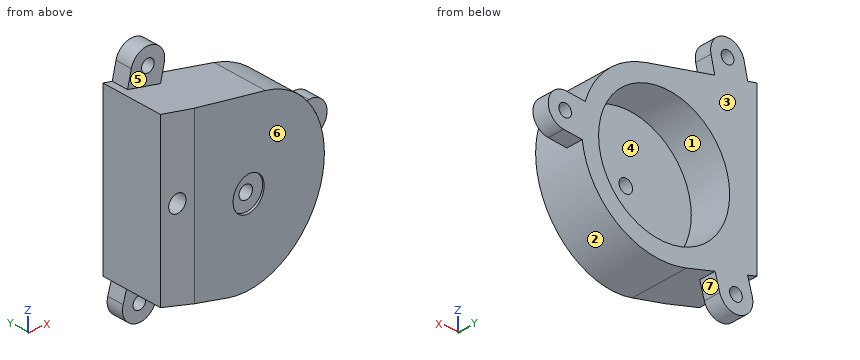
```python
from build123d import *

# Parameters (mm, degrees)
SKETCH1_R               = 15.5
BOSS_EXTRUDE1_DEPTH     = 5
SKETCH2_R               = 15.5
BOSS_EXTRUDE2_DEPTH     = 15
CUT_EXTRUDE7_DEPTH      = 26
CUT_EXTRUDE7_DEPTH_BACK = 20.5
SKETCH18_R              = 1.6
CUT_EXTRUDE8_DEPTH      = 6
SKETCH19_R              = 2.05
CUT_EXTRUDE9_DEPTH      = 6
CUT_EXTRUDE10_REACH     = 4
SKETCH20_R              = 4
SKETCH21_R              = 1.5
SKETCH21_R_2            = 4
BOSS_EXTRUDE3_DEPTH     = 4


with BuildPart() as part:
    # Sketch1 → Boss-Extrude1 (new body)
    with BuildSketch(Plane(origin=(0, 0, 0), x_dir=(1, 0, 0), z_dir=(0, 1, 0))):
        Circle(SKETCH1_R)
    extrude(amount=BOSS_EXTRUDE1_DEPTH)

    # Sketch2 → Boss-Extrude2 (add)
    with BuildSketch(Plane.XZ):
        with BuildLine():
            Line((-22, -14), (-5.351429285, -18.751325409))
            ThreePointArc((-5.351429285, -18.751325409), (18.889988887, -4.839247858), (4.323483194, 19.014665211))
            Line((4.323483194, 19.014665211), (-22, 25))
            Line((-22, 25), (-22, -14))
        make_face()
        Circle(SKETCH2_R, mode=Mode.SUBTRACT)
    extrude(amount=-BOSS_EXTRUDE2_DEPTH)

    # Sketch17 → Cut-Extrude7 (cut, two sides)
    with BuildSketch(Plane.XY) as cut_extrude7_sk:
        Polygon((19.5, 0), (-14, 0), (19.5, 3), align=None)
    extrude(amount=CUT_EXTRUDE7_DEPTH, mode=Mode.SUBTRACT)
    extrude(cut_extrude7_sk.sketch, amount=-CUT_EXTRUDE7_DEPTH_BACK, mode=Mode.SUBTRACT)

    # Sketch18 → Cut-Extrude8 (cut, through all)
    with BuildSketch(Plane(origin=(0, 5, 0), x_dir=(1, 0, 0), z_dir=(0, 1, 0))):
        Circle(SKETCH18_R)
    extrude(amount=-CUT_EXTRUDE8_DEPTH, mode=Mode.SUBTRACT)

    # Sketch19 → Cut-Extrude9 (cut)
    with BuildSketch(Plane.XZ):
        with Locations((-18, 5.5)):
            Circle(SKETCH19_R)
    extrude(amount=-CUT_EXTRUDE9_DEPTH, mode=Mode.SUBTRACT)

    # Sketch20 → Cut-Extrude10 (cut, up to next)
    with BuildSketch(Plane(origin=(0, 2, 0), x_dir=(1, 0, 0), z_dir=(0, 1, 0)), mode=Mode.PRIVATE) as cut_extrude10_sk1:
        Circle(SKETCH20_R)
    cut_extrude10_tool1 = extrude(cut_extrude10_sk1.sketch, amount=-CUT_EXTRUDE10_REACH, mode=Mode.PRIVATE) & part.part
    add(cut_extrude10_tool1.solids().sort_by_distance((0, 2, 0))[0], mode=Mode.SUBTRACT)

    # Sketch21 → Boss-Extrude3 (add)
    with BuildSketch(Plane(origin=(0, 15, 0), x_dir=(1, 0, 0), z_dir=(0, 1, 0))):
        with BuildLine():
            ThreePointArc((-13.153574275, 20.684381981), (-18.097729084, 23.433078622), (-20.846425725, 18.488923813))
            Line((-20.846425725, 18.488923813), (-19.748696641, 14.642498088))
            Line((-19.748696641, 14.642498088), (-12.055845191, 16.837956256))
            Line((-12.055845191, 16.837956256), (-13.153574275, 20.684381981))
        make_face()
        with Locations((-17, 19.586652897)):
            Circle(SKETCH21_R, mode=Mode.SUBTRACT)
        with BuildLine():
            Line((-11.099555854, -26.623594872), (-11.986424202, -22.723150726))
            Line((-11.986424202, -22.723150726), (-19.787312493, -24.496887421))
            Line((-19.787312493, -24.496887421), (-18.900444146, -28.397331567))
            ThreePointArc((-18.900444146, -28.397331567), (-14.113131653, -31.410907365), (-11.099555854, -26.623594872))
        make_face()
        with Locations((-15, -27.51046322)):
            Circle(SKETCH21_R, mode=Mode.SUBTRACT)
        with BuildLine():
            ThreePointArc((23.061952434, -6.032938747), (20.346397625, -4.619310384), (19.425796615, -1.699536959))
            ThreePointArc((19.425796615, -1.699536959), (19.147003171, -3.69354431), (18.664086253, -5.648175312))
            Line((18.664086253, -5.648175312), (23.061952434, -6.032938747))
        make_face()
        with Locations((23.410575405, -2.048159955)):
            Circle(SKETCH21_R_2)
        with Locations((23.410575405, -2.048159955)):
            Circle(SKETCH21_R, mode=Mode.SUBTRACT)
        with BuildLine():
            Line((23.759198376, 1.936618838), (19.361332194, 2.321382272))
            ThreePointArc((19.361332194, 2.321382272), (19.497494408, 0.31258889), (19.425796615, -1.699536959))
            ThreePointArc((19.425796615, -1.699536959), (20.839424976, 1.016017826), (23.759198376, 1.936618838))
        make_face()
    extrude(amount=-BOSS_EXTRUDE3_DEPTH)


solid = part.part
```
The model under review builds one solid part; all positions refer to its coordinate system, in mm. Face numbers are marked on the shaded views. A direction names the side the tool comes from. Give positions to 0.01 mm unless a question says otherwise; leave off trailing zeros. Write each loop counter-clockwise with the first axis right and the second up, starting at its lowest first coordinate (ties: lowest second). Pieces come first, ordered by that corner, then holes.
(1) The part is to be moulded in two halves that separate along Z. For the marked faces 1, 2, 3 and 4, say which applies: released by +Z, released by -Z, zero draft, split by the parting line, or undercut.
(2) To check wall thickness, follow L1, parallel to X at y = 13.25, z = 2; L2, parallel to X at y = 10.5, z = -3; L3, parallel to Z at x = 0, y = 3.35. State the ranges of each line that lie inside material, in increasing order.
(3) Consider section A-A, the plane y = 7.25. Give the boundary of the cut face in (x, z), and give its area (3 significant figures).
(4) Consider section C-C, the plane x = 3. Give the boundary of the cut face in (y, z), and give its area (3 significant figures).
(5) Tool access review of the marked faces 5, 6 and 7: name each direction out of +Z, -Z, +X, -X, +Y, -Y from which nothing blocks a thin tool from reaching the whole face with its end or side.
(6) Consider section B-B, the plane y = 3.75. Give the boundary of the cut face in (x, z).
(7) Consider section D-D, the plane x = 8.5. Give the boundary of the cut face in (y, z), and give its area (3 significant figures).
(8) For P1, Ø3, axis at x = 11.5, z = 19.5, coming from the +Y side; P2, Ø1, axis at x = 10.5, y = 5, coming from the +Z side; P3, Ø4, axis at x = 0, z = 0, coming from the -Y side; P4, Ø4, axis at x = 18, y = 2, coming from the -Z side, all flat-tipped, find the tip position at first contact; note any pin that passes through.
Returned:
1. face 1: undercut
1. face 2: split by the parting line
1. face 3: zero draft
1. face 4: undercut
2. L1: x = -22 to -15.37, 15.37 to 21.91, 24.91 to 27.41
2. L2: x = -22 to -15.21, 15.21 to 19.27
2. L3: z = -19.5 to -1.6, 1.6 to 20
3. outline: (-22, -14) - (-5.35, -18.75) arc R19.5 ccw (long way) to (4.32, 19.01) - (-22, 25) - close; hole circle Ø31 at (0, 0)
3. area: 714 mm2
4. outline: (1.52, -19.27) - (15, -19.27) - (15, -15.21) - (5, -15.21) - (5, 15.21) - (15, 15.21) - (15, 19.32) - (1.52, 19.32) - (1.52, 2.65) - (2, 2.65) - (2, -2.65) - (1.52, -2.65) - close
4. area: 213 mm2
5. face 5: +Z, +X, -Y
5. face 6: +Z, -Z, +X, -Y
5. face 7: -Z, +Y, -Y
6. outline: (-22, -14) - (-5.35, -18.75) arc R19.5 ccw (long way) to (4.32, 19.01) - (-22, 25) - close; hole circle Ø4.1 at (-18, 5.5); hole circle Ø3.2 at (0, 0)
7. outline: (2.01, -17.55) - (15, -17.55) - (15, -12.96) - (5, -12.96) - (5, 12.96) - (15, 12.96) - (15, 17.55) - (2.01, 17.55) - close
7. area: 197 mm2
8. P1: passes through
8. P2: stops at z = 16.74
8. P3: stops at y = 2
8. P4: stops at z = -10.96
